Verification items for the finished model (mm, model axes). Coordinates: 2 decimals unless noted, no trailing zeros. Order: outer loops, then holes, each group sorted by start corner. A loop starts at its lowest first (then second) coordinate and runs counter-clockwise, first axis right, second up. Notation, with made-up numbers: M -22,-16.5 L 18,-16.5 A22 ccw 18,0.5 Z; hole C 36,7 d4. An arc over 180 degrees is marked long. Return JSON: item names as keys, results as strings. Group by question number.
1. Section check B-B, the plane y = 77.5. Record the cut outline in (x, z), plus the area to 3 significant figures.
2. Material ranges on line 1 along Y through (x, z) = (198, -260.5); line 2 along Y through (x, z) = (82, -226), recorded low to high.
3. Section check C-C, the plane x = 263. Record the cut outline in (y, z), plus the area to 3 significant figures.
4. Gauge pin test, flat end, axial feed: pin 1 (1 mm diameter, centred on x = 167.5, z = -222.5, fed in from +Y). Record the tip position at first contact, or that the pin passes through.
5. Section check A-A, the plane z = -150. Record the cut outline in (x, y), plus the area to 3 significant figures.
6. Section check D-D, the plane z = -245. Record the cut outline in (x, y), plus the area to 3 significant figures.
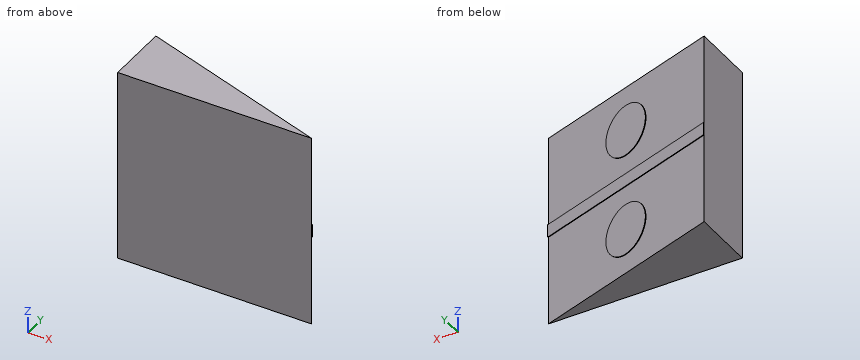
```python
from build123d import *

# Parameters (mm, degrees)
EXTRUDE_1_DEPTH = 300
SKETCH_3_W      = 315.912962697
SKETCH_3_H      = 20
EXTRUDE_2_DEPTH = 1
SKETCH_5_R      = 40
EXTRUDE_3_DEPTH = 1
SKETCH_6_R      = 40
EXTRUDE_4_DEPTH = 1


with BuildPart() as part:
    # Sketch 1 → Extrude 1 (new body)
    with BuildSketch(Plane.XY):
        Polygon((0, 0), (300, 0), (0, 99), align=None)
    extrude(amount=-EXTRUDE_1_DEPTH)

    # Sketch 3 → Extrude 2 (add)
    with BuildSketch(Plane(origin=(29.461628641, 89.277662548, 0), x_dir=(0.9496286491027329, -0.3133774542039019, 0), z_dir=(0.3133774542039019, 0.9496286491027329, 0))):
        with Locations((126.932113383, 150)):
            Rectangle(SKETCH_3_W, SKETCH_3_H)
    extrude(amount=EXTRUDE_2_DEPTH)

    # Sketch 5 → Extrude 3 (add)
    with BuildSketch(Plane(origin=(29.461628641, 89.277662548, 0), x_dir=(0.9496286491027329, -0.3133774542039019, 0), z_dir=(0.3133774542039019, 0.9496286491027329, 0))):
        with Locations(Location((126.932113382, 70, 0), (0, 0, 180))):
            Circle(SKETCH_5_R)
    extrude(amount=EXTRUDE_3_DEPTH)

    # Sketch 6 → Extrude 4 (add)
    with BuildSketch(Plane(origin=(29.461628641, 89.277662548, 0), x_dir=(0.9496286491027329, -0.3133774542039019, 0), z_dir=(0.3133774542039019, 0.9496286491027329, 0))):
        with Locations(Location((126.932113382, 230, 0), (0, 0, 180))):
            Circle(SKETCH_6_R)
    extrude(amount=EXTRUDE_4_DEPTH)


solid = part.part
```
Answers follow:
{
 "1": {"outline": "M 0,-300 L 65.15,-300 L 65.15,-160 L 68.34,-160 L 68.34,-140 L 65.15,-140 L 65.15,0 L 0,0 Z", "area": "19,600 mm^2"},
 "2": {"line 1": "0 to 33.66", "line 2": "0 to 71.94"},
 "3": {"outline": "M 0,-300 L 12.21,-300 L 12.21,-160 L 13.26,-160 L 13.26,-140 L 12.21,-140 L 12.21,0 L 0,0 Z", "area": "3,680 mm^2"},
 "4": {"pin 1": "y = 44.94"},
 "5": {"outline": "M 0,0 L 300,0 L 300.31,0.95 L 0.31,99.95 L 0,99 Z", "area": "15,200 mm^2"},
 "6": {"outline": "M 0,0 L 300,0 L 185.21,37.88 L 185.53,38.83 L 115.1,62.07 L 114.79,61.12 L 0,99 Z", "area": "14,900 mm^2"}
}
